The listing builds one solid part. Answer for the finished solid, in the listing's coordinates (mm). A direction names the side the tool comes from. Coordinates: 2 decimals unless noted, no trailing zeros. Order: outer loops, then holes, each group sorted by start corner. A loop starts at its lowest first (then second) coordinate and runs counter-clockwise, first axis right, second up. Notation, with made-up numbers: (9, 69) -> (66, 69) arc R28 cw to (66, 91) -> close; hole circle Ø4 at (17.25, 61.5). An arc over 180 degrees is marked (long way). One line per question, with ' | ' between items.
from build123d import *

# Parameters (mm, degrees)
SKETCH1_R           = 3.5
BOSS_EXTRUDE1_DEPTH = 8


with BuildPart() as part:
    # Sketch1 → Boss-Extrude1 (new body)
    with BuildSketch(Plane.XY):
        Polygon((25, 0), (-25, 0), (-25, 37), (-22.5, 37), (-22.5, 34), (-18, 34), (-18, 31), (-13.5, 31), (-13.5, 28), (-9, 28), (-9, 25), (-4.5, 25), (-4.5, 22), (4.5, 22), (4.5, 25), (9, 25), (9, 28), (13.5, 28), (13.5, 31), (18, 31), (18, 34), (22.5, 34), (22.5, 37), (25, 37), align=None)
        with Locations((-15, 8)):
            Circle(SKETCH1_R, mode=Mode.SUBTRACT)
        with Locations((15, 8)):
            Circle(SKETCH1_R, mode=Mode.SUBTRACT)
    extrude(amount=BOSS_EXTRUDE1_DEPTH)


solid = part.part
Item 1: Section C-C, the plane z = 6.5 is taken. Give the vertices of the cut face in (x, y), plus the area to 3 significant figures.
Computed values:
outline: (-25, 0) -> (25, 0) -> (25, 37) -> (22.5, 37) -> (22.5, 34) -> (18, 34) -> (18, 31) -> (13.5, 31) -> (13.5, 28) -> (9, 28) -> (9, 25) -> (4.5, 25) -> (4.5, 22) -> (-4.5, 22) -> (-4.5, 25) -> (-9, 25) -> (-9, 28) -> (-13.5, 28) -> (-13.5, 31) -> (-18, 31) -> (-18, 34) -> (-22.5, 34) -> (-22.5, 37) -> (-25, 37) -> close; hole circle Ø7 at (-15, 8); hole circle Ø7 at (15, 8) | area: 1,370 mm^2
Item 2: Each of these flat-tipped pins is pushed along its axis until it touches: pin 1 Ø1.3 at (x, z) = (-20, 2) entering from +Y; pin 2 Ø3.5 at (x, z) = (7, 6) entering from +Y; pin 3 Ø3.5 at (x, z) = (-12, 6) entering from +Y. Where does it stop, or does it pass through?
Computed values:
pin 1: stops at y = 34 | pin 2: stops at y = 25 | pin 3: stops at y = 31
Item 3: For faces 1 (the face through (4.5, 23, 4)), 2 (the face through (0, 15, 8)), determine the directions among +Z, -Z, +X, -X, +Y, -Y from which every point of the face is accessible in a straight line to the end or side of a thin tool.
Computed values:
face 1: +Z, -Z, +Y | face 2: +Z, +X, -X, +Y, -Y
Item 4: Section B-B, the plane y = 23 is taken. Give the vertices of the cut face in (x, z).
Computed values:
outline: (-25, 0) -> (-4.5, 0) -> (-4.5, 8) -> (-25, 8) -> close; (4.5, 0) -> (25, 0) -> (25, 8) -> (4.5, 8) -> close
Item 5: Find the intervals of material crossed by L1, parallel to Y at x = -15, z = 2; L2, parallel to X at y = 31.5, z = 7.5; L3, parallel to X at y = 5.5, z = 7.5, in increasing order.
Computed values:
L1: y = 0 to 4.5, 11.5 to 31 | L2: x = -25 to -18, 18 to 25 | L3: x = -25 to -17.45, -12.55 to 12.55, 17.45 to 25
Item 6: Section D-D, the plane y = 8 is taken. Give the vertices of the cut face in (x, z).
Computed values:
outline: (-25, 0) -> (-18.5, 0) -> (-18.5, 8) -> (-25, 8) -> close; (-11.5, 0) -> (11.5, 0) -> (11.5, 8) -> (-11.5, 8) -> close; (18.5, 0) -> (25, 0) -> (25, 8) -> (18.5, 8) -> close
Item 7: Determine the mould class of faces 3 (the face through (-7, 25, 4)), 4 (the face through (-9, 27, 4)), 5 (the face through (18.233, 6.659, 3.944)) for opening direction Y: pulls with the +Y half, pulls with the -Y half, needs draft (parallel to the pull), parting line crosses it, or undercut.
Computed values:
face 3: pulls with the +Y half | face 4: needs draft | face 5: undercut
Item 8: Section A-A, the plane x = -15 is taken. Give the vertices of the cut face in (y, z).
Computed values:
outline: (0, 0) -> (4.5, 0) -> (4.5, 8) -> (0, 8) -> close; (11.5, 0) -> (31, 0) -> (31, 8) -> (11.5, 8) -> close
